Read the model definition and answer for the solid it produces. Units are mm, in the model's axes. Give positions to 0.01 mm unless a question says otherwise; leave off trailing zeros. Order: outer loops, then holes, each group sorted by start corner. A loop starts at its lowest first (then second) coordinate and runs counter-clockwise, first axis right, second up. Notation, with made-up numbers: (-12.5, 67.25) - (43.5, 67.25) arc R20 ccw to (43.5, 87.25) - close; hole circle Ø11 at (83.5, 58.5). An arc over 180 degrees is marked (long way). Answer as CSV lines item,"result". Start each with the question number.
from build123d import *

# Parameters (mm, degrees)
SKETCH2_W           = 80
SKETCH2_H           = 206.85
BOSS_EXTRUDE1_DEPTH = 3.175
SKETCH3_R           = 2.2
SKETCH3_W           = 20
SKETCH3_H           = 3.175
CUT_EXTRUDE1_DEPTH  = 4.175
FILLET1_R           = 1


with BuildPart() as part:
    # Sketch2 → Boss-Extrude1 (new body)
    with BuildSketch(Plane(origin=(0, 0, 0), x_dir=(1, 0, 0), z_dir=(0, 1, 0))):
        Rectangle(SKETCH2_W, SKETCH2_H)
    extrude(amount=BOSS_EXTRUDE1_DEPTH)

    # Sketch3 → Cut-Extrude1 (cut, through all)
    with BuildSketch(Plane(origin=(0, 3.175, 0), x_dir=(1, 0, 0), z_dir=(0, 1, 0))):
        with Locations((28, 55.882836501)):
            Circle(SKETCH3_R)
        with Locations((-28, 55.882836501)):
            Circle(SKETCH3_R)
        with Locations((0, 87.470336501)):
            Rectangle(SKETCH3_W, SKETCH3_H)
    extrude(amount=-CUT_EXTRUDE1_DEPTH, mode=Mode.SUBTRACT)

    # Fillet1
    fillet1_edges = [part.edges().sort_by_distance(p)[0] for p in [
        (10, 1.5875, -89.057836501),
        (10, 1.5875, -85.882836501),
        (-10, 1.5875, -85.882836501),
        (-10, 1.5875, -89.057836501),
    ]]
    fillet(fillet1_edges, radius=FILLET1_R)


solid = part.part
(1) Straight lines are drawn through the part: line 1 (Z direction, x = -28, y = 1.65) (3 decimals); line 2 (X direction, y = 2.55, z = -87); line 3 (Z direction, x = 27.5, y = 1.55) (3 decimals). For each, find the intervals that lie inside material, in ascending order. Write a range as [from, to].
(2) Section B-B, the plane x = -4 is taken. Write down the section's boundary in (y, z) (3 decimals).
(3) Section A-A, the plane x = 28 is taken. Write down the section's boundary in (y, z) (3 decimals), and give its area (3 significant figures).
(4) Determine the mould class of faces 1 (the flat face through (-1, 3.175, -1)), 2 (the cylindrical face through (27.714, 1.61, -58.064)) for opening direction Z: released by +Z, released by -Z, zero draft, split by the parting line, or undercut.
Checks:
1,line 1,"z = [-103.425, -58.083], [-53.683, 103.425]"
1,line 2,"x = [-40, -10], [10, 40]"
1,line 3,"z = [-103.425, -58.025], [-53.74, 103.425]"
2,outline,"(0, -103.425) - (3.175, -103.425) - (3.175, -89.058) - (0, -89.058) - close; (0, -85.883) - (3.175, -85.883) - (3.175, 103.425) - (0, 103.425) - close"
3,outline,"(0, -103.425) - (3.175, -103.425) - (3.175, -58.083) - (0, -58.083) - close; (0, -53.683) - (3.175, -53.683) - (3.175, 103.425) - (0, 103.425) - close"
3,area,"643 mm²"
4,face 1,"zero draft"
4,face 2,"undercut"
